from build123d import *

# Parameters (mm, degrees)
SKETCH11_R               = 8
BOSS_EXTRUDE5_DEPTH      = 15.5
SKETCH12_R               = 2.5
CUT_EXTRUDE9_DEPTH       = 20.189841062
CUT_EXTRUDE11_START      = -7.4
SKETCH14_R               = 8
SKETCH14_R_2             = 5.8
CUT_EXTRUDE11_DEPTH      = 7.4
CUT_EXTRUDE12_DEPTH      = 7.4
CIRPATTERN5_COUNT        = 20
SKETCH16_R               = 8
BOSS_EXTRUDE6_DEPTH      = 0.5
SKETCH17_R               = 2.5
CUT_EXTRUDE13_DEPTH      = 20.189841062
CUT_EXTRUDE14_REACH      = 21.596
CUT_EXTRUDE14_END_RADIUS = 8
SKETCH18_R               = 2
CIRPATTERN6_COUNT        = 3


with BuildPart() as part:
    # Sketch11 → Boss-Extrude5 (new body)
    with BuildSketch(Plane(origin=(0, 0, 0), x_dir=(1, 0, 0), z_dir=(0, 1, 0))):
        with Locations(Location((0, 0, 0), (0, 0, 270))):
            Circle(SKETCH11_R)
    extrude(amount=BOSS_EXTRUDE5_DEPTH)

    # Sketch12 → Cut-Extrude9 (cut, through all)
    with BuildSketch(Plane(origin=(0, 15.5, 0), x_dir=(1, 0, 0), z_dir=(0, 1, 0))):
        with Locations(Location((0, 0, 0), (0, 0, 270))):
            Circle(SKETCH12_R)
    extrude(amount=-CUT_EXTRUDE9_DEPTH, mode=Mode.SUBTRACT)

    # Sketch14 → Cut-Extrude11 (cut)
    with BuildSketch(Plane(origin=(0, 15.5, 0), x_dir=(1, 0, 0), z_dir=(0, 1, 0)).offset(CUT_EXTRUDE11_START)):
        with Locations(Location((0, 0, 0), (0, 0, 270))):
            Circle(SKETCH14_R)
        with Locations(Location((0, 0, 0), (0, 0, 270))):
            Circle(SKETCH14_R_2, mode=Mode.SUBTRACT)
    extrude(amount=CUT_EXTRUDE11_DEPTH, mode=Mode.SUBTRACT)

    # Sketch15 → Cut-Extrude12 (cut)
    with BuildSketch(Plane(origin=(0, 15.5, 0), x_dir=(1, 0, 0), z_dir=(0, 1, 0))):
        Polygon((-0.75, 5.8), (0.75, 5.8), (0.25, 4.3), (-0.25, 4.3), align=None)
    cut_extrude12 = extrude(amount=-CUT_EXTRUDE12_DEPTH, mode=Mode.SUBTRACT)

    # CirPattern5: Cut-Extrude12 ×20 about axis
    cirpattern5_axis = Axis((0, 0, 0), (0, 1, 0))
    for i in range(1, CIRPATTERN5_COUNT):
        add(cut_extrude12.rotate(cirpattern5_axis, i * 360 / CIRPATTERN5_COUNT), mode=Mode.SUBTRACT)

    # Sketch16 → Boss-Extrude6 (add)
    with BuildSketch(Plane(origin=(0, 15.5, 0), x_dir=(1, 0, 0), z_dir=(0, 1, 0))):
        with Locations(Location((0, 0, 0), (0, 0, 270))):
            Circle(SKETCH16_R)
    extrude(amount=BOSS_EXTRUDE6_DEPTH)

    # Sketch17 → Cut-Extrude13 (cut, through all)
    with BuildSketch(Plane.XZ.offset(-15.5)):
        with Locations(Location((0, 0, 0), (0, 0, 90))):
            Circle(SKETCH17_R)
    extrude(amount=-CUT_EXTRUDE13_DEPTH, mode=Mode.SUBTRACT)

    # Cut-Extrude14: up to this cylinder (the profile starts inside it)
    cut_extrude14_end = Plane(origin=(0, 4, 0), z_dir=(0, -1, 0)) * Cylinder(CUT_EXTRUDE14_END_RADIUS, 60.192, mode=Mode.PRIVATE)
    # Sketch18 → Cut-Extrude14 (cut, up to the surface)
    with BuildSketch(Plane.XY, mode=Mode.PRIVATE) as cut_extrude14_sk1:
        with Locations((0, 4)):
            Circle(SKETCH18_R)
    cut_extrude14_tool1 = extrude(cut_extrude14_sk1.sketch, amount=-CUT_EXTRUDE14_REACH, mode=Mode.PRIVATE) & cut_extrude14_end
    cut_extrude14 = cut_extrude14_tool1.solids().sort_by_distance((0, 4, 0))[0]
    add(cut_extrude14, mode=Mode.SUBTRACT)

    # CirPattern6: Cut-Extrude14 ×3 about axis
    cirpattern6_axis = Axis((0, 0, 0), (0, 1, 0))
    for i in range(1, CIRPATTERN6_COUNT):
        add(cut_extrude14.rotate(cirpattern6_axis, i * 360 / CIRPATTERN6_COUNT), mode=Mode.SUBTRACT)


solid = part.part
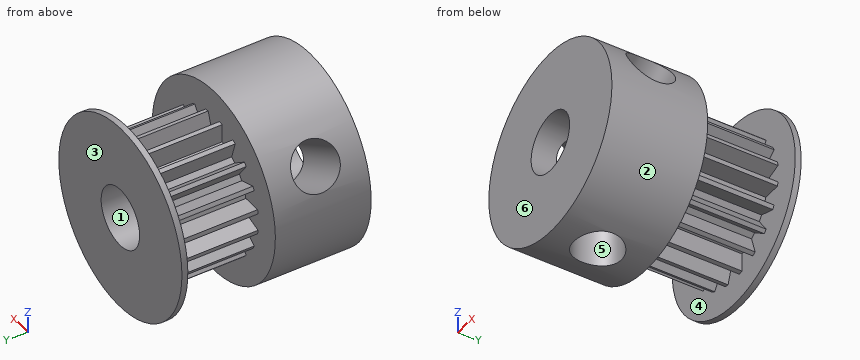
The listing builds one solid part. Answer for the finished solid, in the listing's coordinates (mm). Face numbers are marked on the shaded views. A direction names the side the tool comes from. Coordinates: 2 decimals unless noted, no trailing zeros. Loops run counter-clockwise (first coordinate to the right, second up) from the corner with the lowest first, then second, coordinate; pieces in that order, holes last. Notation, with made-up numbers: M 21,85.5 L 73,85.5 A20 cw 73,124.5 Z; hole C 19.25,41.25 d5. An arc over 180 degrees is marked long. Answer in a Markdown table with one row per item.
1) Find section A-A (x = 0). Determine the outline of the cut face in (y, z).
Answers below:
| item | result |
|---|---|
| outline | M 0,-8 L 2,-8 L 2,-2.5 L 0,-2.5 Z; M 0,2.5 L 16,2.5 L 16,8 L 15.5,8 L 15.5,4.3 L 8.1,4.3 L 8.1,8 L 0,8 Z; M 6,-8 L 8.1,-8 L 8.1,-4.3 L 15.5,-4.3 L 15.5,-8 L 16,-8 L 16,-2.5 L 6,-2.5 Z |
2) Find section C-C (z = -2). Determine the outline of the cut face in (x, y), then the cut area to 3 significant figures.
Answers below:
| item | result |
|---|---|
| outline | M -7.75,0 L -1.5,0 L -1.5,2.68 A2 cw -1.5,5.32 L -1.5,16 L -7.75,16 L -7.75,15.5 L -4.6,15.5 L -4.6,8.1 L -7.75,8.1 Z; M 1.5,0 L 7.75,0 L 7.75,8.1 L 4.6,8.1 L 4.6,15.5 L 7.75,15.5 L 7.75,16 L 1.5,16 L 1.5,5.32 A2 cw 1.5,2.68 Z |
| area | 151 mm^2 |
3) Find section B-B (y = 4). Determine the outline of the cut face in (x, z).
Answers below:
| item | result |
|---|---|
| outline | M -7.71,2.14 A8 ccw -2,-7.75 L -2,-1.5 A2.5 cw -2.3,-0.98 Z; M -5.71,5.61 L -0.3,2.48 A2.5 cw 0.3,2.48 L 5.71,5.61 A8 ccw Z; M 2,-7.75 A8 ccw 7.71,2.14 L 2.3,-0.98 A2.5 cw 2,-1.5 Z |
4) Which of the six approach directions +Z, -Z, +X, -X, +Y, -Y give full straight-line access (tool end or side, diameter ignored) to the marked faces 4, 5 and 6?
Answers below:
| item | result |
|---|---|
| face 4 | none |
| face 5 | -Z |
| face 6 | +Z, -Z, +X, -X, -Y |
5) Find section D-D (z = 4.75). Count the separate pieces of the cut face and the enclosed holes in it, then the cut area to 3 significant figures.
Answers below:
| item | result |
|---|---|
| separate pieces | 1 |
| enclosed holes | 3 |
| area | 118 mm^2 |
6) Determine the mould class of the marked faces 1, 2 and 3 for opening direction Z: released by +Z, released by -Z, zero draft, split by the parting line, or undercut.
Answers below:
| item | result |
|---|---|
| face 1 | undercut |
| face 2 | split by the parting line |
| face 3 | zero draft |
7) Given pin 1 (5 mm diameter, centred on y = 5.5, z = -3.5, fed in from -X); pin 2 (6 mm diameter, centred on y = 5, z = -2.5, fed in from +X); pin 3 (5 mm diameter, centred on y = 12.5, z = -5.5, fed in from -X); pin 4 (4 mm diameter, centred on y = 14.5, z = 6, fed in from +X), each flat-ended and moving along its own axis, determine where each tip first touches the part or whether it passes through.
Answers below:
| item | result |
|---|---|
| pin 1 | x = -7.94 |
| pin 2 | x = 8 |
| pin 3 | x = -4.22 |
| pin 4 | x = 6.77 |
8) Find the intervals of material crossed by probe 1 along Y at (x, z) = (6, -4.75); probe 2 along X at (y, z) = (6, 0); probe 3 along Z at (x, y) = (0, 9.5), in increasing order.
Answers below:
| item | result |
|---|---|
| probe 1 | 0 to 8.1, 15.5 to 16 |
| probe 2 | -8 to -2.5, 2.5 to 8 |
| probe 3 | -4.3 to -2.5, 2.5 to 4.3 |
